Input: part model. Units: mm. Frame: model coordinates. Face numbers are marked on the shaded views. Coordinates: 2 decimals unless noted, no trailing zeros. Order: outer loops, then holes, each group sorted by start corner. A loop starts at its lowest first (then second) coordinate and runs counter-clockwise, first axis right, second up. Notation, with made-up numbers: M 36.5,-34.75 L 95.5,-34.75 A15 cw 95.5,-24.75 Z; hole C -17,15.5 d6. An arc over 180 degrees is marked long. One line per item, written item: value.
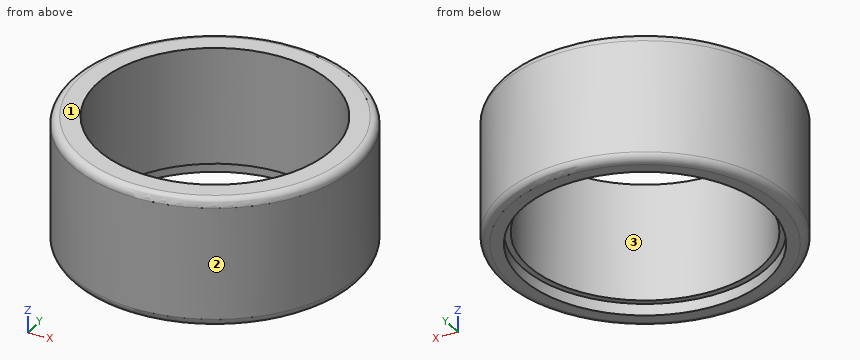
```python
from build123d import *

# Parameters (mm, degrees)
F0_R     = 12.25
F0_R_2   = 10.5
F0_R_3   = 10
F1_DEPTH = 11
F2_DEPTH = 1
F3_R     = 0.7


with BuildPart() as f1:
    # F0 (on Top) → F1 (new body)
    with BuildSketch(Plane.XY):
        Circle(F0_R)
        Circle(F0_R_2, mode=Mode.SUBTRACT)
        Circle(F0_R_2)
        Circle(F0_R_3, mode=Mode.SUBTRACT)
    extrude(amount=F1_DEPTH)

    # F0 (on Top) → F2 (cut)
    with BuildSketch(Plane.XY):
        Circle(F0_R_2)
        Circle(F0_R_3, mode=Mode.SUBTRACT)
    extrude(amount=F2_DEPTH, mode=Mode.SUBTRACT)

    # F3
    f3_edges = [f1.edges().sort_by_distance(p)[0] for p in [
        (-12.25, 0, 0),
        (-12.25, 0, 11),
    ]]
    fillet(f3_edges, radius=F3_R)


solid = f1.part
```
(1) Cut plane C-C on z = 10. Output: boundary loops of the cut face in (x, y), plus the area to 3 significant figures.
Data:
outline: C 0,0 d24.5; hole C 0,0 d20
area: 157 mm2
(2) Draft query along Y for the marked faces 1, 2 and 3. Return one class per face: released by +Y, released by -Y, zero draft, split by the parting line, or undercut.
Data:
face 1: zero draft
face 2: split by the parting line
face 3: undercut
(3) First-contact query: pin 1 (2 mm diameter, centred on y = 7, z = 7.5, fed in from +X); pin 2 (1 mm diameter, centred on y = 1, z = 2.5, fed in from -X); pin 3 (1.5 mm diameter, centred on x = 4, z = 3, fed in from +Y). Flat tips, straight axial feed; report the tip coordinate or a pass-through.
Data:
pin 1: stops at x = 10.68
pin 2: stops at x = -12.24
pin 3: stops at y = 11.81
(4) Cut plane A-A on x = 0. Output: boundary loops of the cut face in (y, z), plus the area to 3 significant figures.
Data:
outline: M -12.25,0.7 A0.7 ccw -11.55,0 L -10.5,0 L -10.5,1 L -10,1 L -10,11 L -11.55,11 A0.7 ccw -12.25,10.3 Z; M 10,1 L 10.5,1 L 10.5,0 L 11.55,0 A0.7 ccw 12.25,0.7 L 12.25,10.3 A0.7 ccw 11.55,11 L 10,11 Z
area: 48.1 mm2
(5) Ray query, line 1 (Y direction, x = 0, z = 0.75); line 2 (Y direction, x = 0, z = 8.5); line 3 (X direction, y = 6.25, z = 9.75). Return the intervals inside material, ascending. Write a range as from..to.
Data:
line 1: y = -12.25..-10.5, 10.5..12.25
line 2: y = -12.25..-10, 10..12.25
line 3: x = -10.54..-7.81, 7.81..10.54
